Answer from the drawing. Dimensions are ordinates in mm from the lowest x, y and z of the part. A direction names the side the tool comes from. Round coordinates to 2 decimals unless told otherwise and drop trailing zeros. Order: outer loops, then holes, each group sorted by start corner. A loop starts at its lowest first (then second) coordinate and runs counter-clockwise, first axis right, second up.
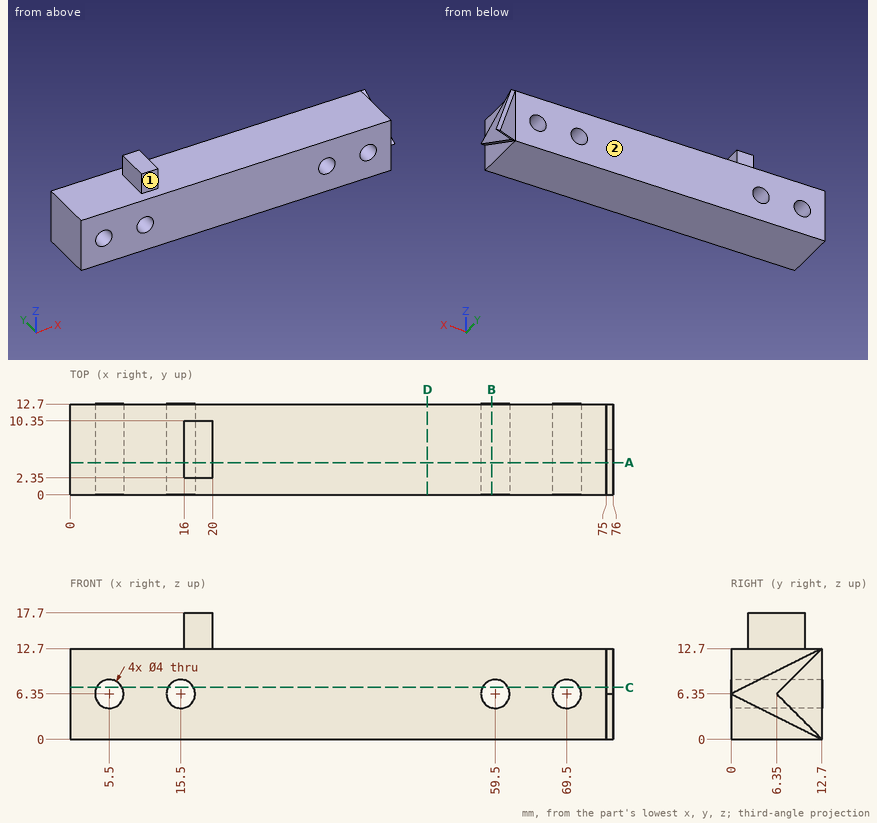
Q1. Straight lines are drawn through the part: probe 1 along Z at (x, y) = (5.5, 8); probe 2 along X at (y, z) = (1, 1.25); probe 3 along Z at (x, y) = (34.5, 9). For each, find the intervals that lie inside material, in ascending order.
Outcome:
probe 1: z = 0 to 4.35, 8.35 to 12.7
probe 2: x = 0 to 75
probe 3: z = 0 to 12.7
Q2. A cutting plane is placed at A-A, the plane y = 4.5. Give the vertices of the cut face in (x, z), plus the area to 3 significant figures.
Outcome:
outline: (0, 0) - (75, 0) - (75, 4.1) - (76, 4.1) - (76, 8.6) - (75, 8.6) - (75, 12.7) - (20, 12.7) - (20, 17.7) - (16, 17.7) - (16, 12.7) - (0, 12.7) - close; hole circle Ø4 at (5.5, 6.35); hole circle Ø4 at (15.5, 6.35); hole circle Ø4 at (59.5, 6.35); hole circle Ø4 at (69.5, 6.35)
area: 927 mm2
Q3. A cutting plane is placed at B-B, the plane x = 59. Give the vertices of the cut face in (y, z).
Outcome:
outline: (0, 0) - (12.7, 0) - (12.7, 4.41) - (0, 4.41) - close; (0, 8.29) - (12.7, 8.29) - (12.7, 12.7) - (0, 12.7) - close
Q4. For the marked faces 1 and 2, determine the directions among +Z, -Z, +X, -X, +Y, -Y from which every point of the face is accessible in a straight line to the end or side of a thin tool.
Outcome:
face 1: +Z, +X, -X, -Y
face 2: +Z, -Z, +X, -X, +Y
Q5. A cutting plane is placed at D-D, the plane x = 50. Give the vertices of the cut face in (y, z).
Outcome:
outline: (0, 0) - (12.7, 0) - (12.7, 12.7) - (0, 12.7) - close
Q6. Flat-ended cylindrical pins translate along their axes: pin 1 (3.5 mm diameter, centred on x = 5.5, z = 6.35, fed in from +Y) (1 decimal); pin 2 (1.5 mm diameter, centred on y = 5.5, z = 14, fed in from +X); pin 3 (3 mm diameter, centred on x = 17, z = 14.5, fed in from +Y); pin 4 (5.5 mm diameter, centred on y = 5.5, z = 15.5, fed in from -X). Find the tip coordinate at first contact, or state that the pin passes through.
Outcome:
pin 1: passes through
pin 2: stops at x = 20
pin 3: stops at y = 10.35
pin 4: stops at x = 16
Q7. A cutting plane is placed at C-C, the plane z = 7.25. Give the vertices of the cut face in (x, y), plus the area to 3 significant figures.
Outcome:
outline: (0, 0) - (3.71, 0) - (3.71, 12.7) - (0, 12.7) - close; (7.29, 0) - (13.71, 0) - (13.71, 12.7) - (7.29, 12.7) - close; (17.29, 0) - (57.71, 0) - (57.71, 12.7) - (17.29, 12.7) - close; (61.29, 0) - (67.71, 0) - (67.71, 12.7) - (61.29, 12.7) - close; (71.29, 0) - (75, 0) - (75, 1.8) - (76, 1.8) - (76, 7.25) - (75, 7.25) - (75, 12.7) - (71.29, 12.7) - close
area: 776 mm2
